The listing builds one solid part. Answer for the finished solid, in the listing's coordinates (mm). Face numbers are marked on the shaded views. A direction names the side the tool comes from. Give positions to 0.01 mm unless a question says otherwise; leave off trailing zeros. Order: outer loops, then holes, each group sorted by start corner. A loop starts at its lowest first (then second) coordinate and runs counter-clockwise, first axis right, second up. Notation, with made-up numbers: (15.25, -13.5) - (67.25, -13.5) arc R20 ccw to (67.25, -2.5) - close; hole circle Ø8 at (46.25, -22). An arc over 180 degrees is marked (long way). Answer in a Markdown table with one row per item.
from build123d import *

# Parameters (mm, degrees)
SKETCH2_W         = 8.001
SKETCH2_H         = 8.001
SQUARE_BOSS_DEPTH = 4.445


with BuildPart() as part:
    # Sketch1 → Screw revolve (revolve)
    with BuildSketch(Plane.XY, mode=Mode.PRIVATE) as screw_revolve_sk:
        with BuildLine():
            Line((0, 0), (3.96875, 0))
            Line((3.96875, 0), (3.96875, 19.05))
            Line((3.96875, 19.05), (8.763, 19.05))
            Line((8.763, 19.05), (8.763, 21.082))
            ThreePointArc((8.763, 21.082), (4.497754801, 22.599348829), (0, 23.114))
            Line((0, 23.114), (0, 0))
        make_face()
    revolve(screw_revolve_sk.sketch.rotate(Axis((0, 0, 0), (0, 1, 0)), 90), axis=Axis((0, 0, 0), (0, 1, 0)))

    # Sketch2 → Square boss (add)
    with BuildSketch(Plane.XZ.offset(-19.05)):
        Rectangle(SKETCH2_W, SKETCH2_H)
    extrude(amount=SQUARE_BOSS_DEPTH)


solid = part.part
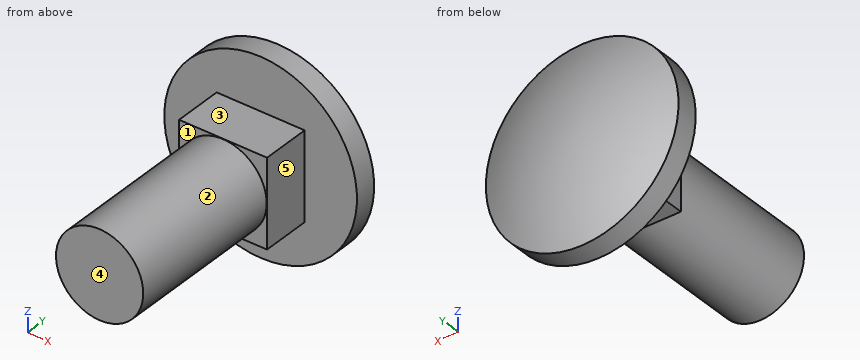
Item 1: Find section C-C on y = 15. Write down the section's boundary in (x, z).
Answer block:
| item | result |
|---|---|
| outline | (-4, -4) - (4, -4) - (4, 4) - (-4, 4) - close |
Item 2: Consider line 1 (X direction, y = 17.5, z = 2.25); line 2 (Y direction, x = -2.25, z = -4.5); line 3 (Z direction, x = 6.25, y = 21). Determine where each line is inside the solid, lowest interval first.
Answer block:
| item | result |
|---|---|
| line 1 | -4 to 4 |
| line 2 | 19.05 to 22.47 |
| line 3 | -6.14 to 6.14 |
Item 3: Find section D-D on y = 4.75. Write down the section's boundary in (x, z), then the cut area to 3 significant figures.
Answer block:
| item | result |
|---|---|
| outline | circle Ø7.94 at (0, 0) |
| area | 49.5 mm² |
Item 4: Which of the six approach directions +Z, -Z, +X, -X, +Y, -Y give full straight-line access (tool end or side, diameter ignored) to the marked faces 4 and 5?
Answer block:
| item | result |
|---|---|
| face 4 | +Z, -Z, +X, -X, -Y |
| face 5 | +Z, -Z, +X, -Y |
Item 5: Determine the mould class of the marked faces 1, 2 and 3 for opening direction Z: pulls with the +Z half, pulls with the -Z half, needs draft (parallel to the pull), parting line crosses it, or undercut.
Answer block:
| item | result |
|---|---|
| face 1 | needs draft |
| face 2 | parting line crosses it |
| face 3 | pulls with the +Z half |
Item 6: Each of these flat-tipped pins is pushed along its axis until it touches: P1, Ø2, axis at x = 3, y = 9, coming from the +Z side; P2, Ø1.3, axis at y = 16, z = 0.5, coming from the +X side; P3, Ø5, axis at x = -2, y = 15.5, coming from the -Z side; P4, Ø1, axis at y = 17, z = 5, coming from the +X side. Where does it stop, or does it pass through?
Answer block:
| item | result |
|---|---|
| P1 | z = 3.43 |
| P2 | x = 4 |
| P3 | z = -4 |
| P4 | through |
